Input: part model. Units: mm. Frame: model coordinates. Coordinates: 2 decimals unless noted, no trailing zeros. Write each loop counter-clockwise with the first axis right and the second up, starting at its lowest first coordinate (ties: lowest second). Pieces come first, ordered by that corner, then holes.
1) Line query: L1, parallel to Z at x = 0.5, y = 3; L2, parallel to X at y = 3.15, z = -1; L3, parallel to X at y = 0.35, z = 10. Output: solid intervals per line, ascending.
2) Section query B-B (z = -15.5). Output: boundary loops of the cut face in (x, y).
3) Section query C-C (y = 2.1). Output: boundary loops of the cut face in (x, z), then the cut area to 3 significant figures.
4) Pin query (flat end, axial travel): pin 1 Ø1.5 at (y, z) = (3, -8.5) entering from +X; pin 2 Ø4 at (x, z) = (-1.5, 6) entering from -Y; pin 3 Ø1.5 at (x, y) = (4.5, 3) entering from +Z. Return the tip coordinate at first contact, or that it passes through.
5) Section query A-A (x = -8.5). Output: boundary loops of the cut face in (y, z), then the cut area to 3 significant figures.
6) Draft query along Z for faces 1 (the flat face through (0, 2, -18.5)), 2 (the cylindrical face through (-9.4, 0.5, 2)), 3 (the flat face through (-10, 0.5, -4)). Return one class per face: pulls with the +Z half, pulls with the -Z half, needs draft (parallel to the pull), parting line crosses it, or undercut.
Autodesk Inventor part; units mm, degrees
ref_plane "YZ Plane" through (0, 0, 0) normal (1, 0, 0) x (0, 1, 0)
ref_plane "XZ Plane" through (0, 0, 0) normal (0, 1, 0) x (-1, 0, 0)
ref_plane "XY Plane" through (0, 0, 0) normal (0, 0, 1) x (1, 0, 0)
sketch "Sketch1" plane through (0, 0, 0) normal (0, 1, 0) x (-1, 0, 0)
  line L0 (-10, 19) -> (10, 19)
  line L1 (10, 19) -> (10, -19)
  line L2 (10, -19) -> (-10, -19)
  line L3 (-10, -19) -> (-10, 19)
  line L4 (-10, 19) -> (10, -19) construction
  line L5 (10, 19) -> (-10, -19) construction
  circle A0 centre (10, 14) radius 0.6
  circle A1 centre (10, 10) radius 0.6
  circle A2 centre (10, 6) radius 0.6
  circle A3 centre (10, 2) radius 0.6
  circle A4 centre (10, -2) radius 0.6
  circle A5 centre (10, -6) radius 0.6
  circle A6 centre (10, -10) radius 0.6
  circle A7 centre (10, -14) radius 0.6
  circle A8 centre (-10, 14) radius 0.6
  circle A9 centre (-10, 10) radius 0.6
  circle A10 centre (-10, 6) radius 0.6
  circle A11 centre (-10, 2) radius 0.6
  circle A12 centre (-10, -2) radius 0.6
  circle A13 centre (-10, -6) radius 0.6
  circle A14 centre (-9.9999, -10) radius 0.6
  circle A15 centre (-9.9999, -14) radius 0.6
  point P0 (0, 0)
  dimension "d0" = 20
  dimension "d1" = 38
  dimension "d2" = 1.2
  dimension "d3" = 0
  dimension "d4" = 5
  dimension "d5" = 1.2
  dimension "d6" = 1.2
  dimension "d7" = 0
  dimension "d8" = 0
  dimension "d9" = 4
  dimension "d10" = 4
  dimension "d11" = 1.2
  dimension "d13" = 1.2
  dimension "d14" = 1.2
  dimension "d15" = 0
  dimension "d16" = 0
  dimension "d17" = 0
  dimension "d18" = 4
  dimension "d19" = 4
  dimension "d20" = 4
  dimension "d22" = 1.2
  dimension "d23" = 0
  dimension "d24" = 4
  dimension "d25" = 1.2
  dimension "d26" = 0
  dimension "d27" = 4
  dimension "d28" = 1.2
  dimension "d29" = 1.2
  dimension "d30" = 1.2
  dimension "d31" = 4
  dimension "d32" = 4
  dimension "d33" = 1.2
  dimension "d34" = 4
  dimension "d35" = 5
  dimension "d36" = 0
  dimension "d37" = 1.2
  dimension "d38" = 1.2
  dimension "d39" = 1.2
  dimension "d40" = 4
  dimension "d41" = 4
  dimension "d42" = 1.2
  dimension "d43" = 4
  dimension "d44" = 5
  dimension "d45" = 0
  dimension "d46" = 4
extrude "Extrusion1" add sketch "Sketch1" along normal blind 1 contours L0 L1 A0 A1 A2 A3 A4 A5 A6 A7 L2 L3 A15 A14 A13 A12 A11 A10 A9 A8 | A8 L3 | L1 A0 | A9 L3 | L1 A1 | A10 L3 | L1 A2 | A11 L3 | L1 A3 | A12 L3 | L1 A4 | A13 L3 | L1 A5 | A14 L3 | L1 A6 | A15 L3 | L1 A7 picked at (-9.7546, 14.1247) picked at (9.9071, 13.8229) picked at (-9.7546, 10.1247) picked at (9.9071, 9.8229) picked at (-9.7991, 6.1197) picked at (9.6869, 6.1942) picked at (-9.7124, 2.1099) picked at (9.9521, 1.8058) picked at (-9.8308, -1.8486) picked at (9.9521, -2.1942) picked at (-9.7863, -5.8436) picked at (9.6325, -6.0264) picked at (-9.8, -10) picked at (9.7266, -9.8332) picked at (-9.8, -14) picked at (9.7266, -13.8332)
sketch "Sketch2" plane through (0, 1, 0) normal (0, 1, 0) x (1, 0, 0)
  line L0 (-10, 19) -> (10, 19)
  line L1 (10, 19) -> (10, -19)
  line L2 (10, -19) -> (-10, -19)
  line L3 (-10, -19) -> (-10, 19)
  line L4 (-10, 19) -> (10, -19) construction
  line L5 (10, 19) -> (-10, -19) construction
  circle A0 centre (10, 14) radius 0.6
  circle A1 centre (10, 10) radius 0.6
  circle A2 centre (10, 6) radius 0.6
  circle A3 centre (10, 2) radius 0.6
  circle A4 centre (10, -2) radius 0.6
  circle A5 centre (10, -6) radius 0.6
  circle A6 centre (10, -10) radius 0.6
  circle A7 centre (10, -14) radius 0.6
  circle A8 centre (-10, 14) radius 0.6
  circle A9 centre (-10, 10) radius 0.6
  circle A10 centre (-10, 6) radius 0.6
  circle A11 centre (-10, 2) radius 0.6
  circle A12 centre (-10, -2) radius 0.6
  circle A13 centre (-10, -6) radius 0.6
  circle A14 centre (-9.9999, -10) radius 0.6
  circle A15 centre (-9.9999, -14) radius 0.6
  point P0 (0, 0)
  point P1 (0, 0)
  dimension "d49" = 20
  dimension "d50" = 38
  dimension "d51" = 1.2
  dimension "d52" = 0
  dimension "d53" = 5
  dimension "d54" = 1.2
  dimension "d55" = 1.2
  dimension "d56" = 0
  dimension "d57" = 0
  dimension "d58" = 4
  dimension "d59" = 4
  dimension "d60" = 1.2
  dimension "d61" = 1.2
  dimension "d62" = 1.2
  dimension "d63" = 0
  dimension "d64" = 0
  dimension "d65" = 0
  dimension "d66" = 4
  dimension "d67" = 4
  dimension "d68" = 4
  dimension "d69" = 1.2
  dimension "d70" = 0
  dimension "d71" = 4
  dimension "d72" = 1.2
  dimension "d73" = 0
  dimension "d74" = 4
  dimension "d75" = 1.2
  dimension "d76" = 1.2
  dimension "d77" = 1.2
  dimension "d78" = 4
  dimension "d79" = 4
  dimension "d80" = 1.2
  dimension "d81" = 4
  dimension "d82" = 5
  dimension "d83" = 0
  dimension "d84" = 1.2
  dimension "d85" = 1.2
  dimension "d86" = 1.2
  dimension "d87" = 4
  dimension "d88" = 4
  dimension "d89" = 1.2
  dimension "d90" = 4
  dimension "d91" = 5
  dimension "d92" = 0
  dimension "d93" = 4
extrude "Extrusion2" cut sketch "Sketch2" against normal blind 1 contours A8 L3 | L3 A8 | A0 L1 | L1 A0 | A9 L3 | L3 A9 | A1 L1 | L1 A1 | A10 L3 | L3 A10 | A2 L1 | L1 A2 | A11 L3 | L3 A11 | A3 L1 | L1 A3 | A12 L3 | L3 A12 | A4 L1 | L1 A4 | A13 L3 | L3 A13 | A5 L1 | L1 A5 | A14 L3 | L3 A14 | A6 L1 | L1 A6 | A15 L3 | L3 A15 | A7 L1 | L1 A7
sketch "Sketch3" plane through (0, 1, 0) normal (0, 1, 0) x (1, 0, 0)
  line L0 (-9, -18.5) -> (9, -18.5)
  line L1 (9, -18.5) -> (9, 18.5)
  line L2 (9, 18.5) -> (-9, 18.5)
  line L3 (-9, 18.5) -> (-9, -18.5)
  line L4 (-9, -18.5) -> (9, 18.5) construction
  line L5 (9, -18.5) -> (-9, 18.5) construction
  point P0 (0, 0)
  dimension "d96" = 37
extrude "Extrusion3" add sketch "Sketch3" along normal blind 3
properties part number "Radio"
Answer:
1. L1: z = -18.5 to 18.5
1. L2: x = -9 to 9
1. L3: x = -9.4 to 9.4
2. outline: (-10, 0) - (10, 0) - (10, 1) - (9, 1) - (9, 4) - (-9, 4) - (-9, 1) - (-10, 1) - close
3. outline: (-9, -18.5) - (9, -18.5) - (9, 18.5) - (-9, 18.5) - close
3. area: 666 mm2
4. pin 1: stops at x = 9
4. pin 2: stops at y = 0
4. pin 3: stops at z = 18.5
5. outline: (0, -19) - (1, -19) - (1, -18.5) - (4, -18.5) - (4, 18.5) - (1, 18.5) - (1, 19) - (0, 19) - close
5. area: 149 mm2
6. face 1: pulls with the -Z half
6. face 2: undercut
6. face 3: needs draft
